Here's how the part is built. I have some questions about the finished solid (model axes, mm). Give positions to 0.01 mm unless a question says otherwise; leave off trailing zeros. Loops run counter-clockwise (first coordinate to the right, second up) from the corner with the lowest first, then second, coordinate; pieces in that order, holes last. Notation, with made-up numbers: (64, 86) - (68, 86) arc R25 ccw to (68, 98) - close; hole circle Ø10 at (28.25, -39.5). An arc over 180 degrees is marked (long way). Use a Markdown table: item, result.
from build123d import *

# Parameters (mm, degrees)
SKETCH1_W                = 50
SKETCH1_H                = 50
BOSS_EXTRUDE1_DEPTH      = 3.175
M3_CLEARANCE_HOLE1_D     = 3.2
M3_CLEARANCE_HOLE1_DEPTH = 12.4
M3_CLEARANCE_HOLE1_TIP   = 0.96137699
M3X0_5_TAPPED_HOLE1_D    = 2.5
FILLET1_R                = 3


with BuildPart() as part:
    # Sketch1 → Boss-Extrude1 (new body)
    with BuildSketch(Plane(origin=(0, 0, 0), x_dir=(1, 0, 0), z_dir=(0, 1, 0))):
        Rectangle(SKETCH1_W, SKETCH1_H)
    extrude(amount=BOSS_EXTRUDE1_DEPTH)

    # M3 Clearance Hole1
    with Locations(Plane(origin=(0, 3.175, 0), x_dir=(1, 0, 0), z_dir=(0, 1, 0))):
        with Locations((-20, 20), (20, 20), (-20, -20), (20, -20)):
            Hole(M3_CLEARANCE_HOLE1_D / 2, depth=M3_CLEARANCE_HOLE1_DEPTH)
            with Locations((0, 0, -(M3_CLEARANCE_HOLE1_DEPTH + M3_CLEARANCE_HOLE1_TIP / 2))):  # 118° drill point
                Cone(0, M3_CLEARANCE_HOLE1_D / 2, M3_CLEARANCE_HOLE1_TIP, mode=Mode.SUBTRACT)

    # M3x0.5 Tapped Hole1 (through all)
    with Locations(Plane(origin=(0, 3.175, 0), x_dir=(1, 0, 0), z_dir=(0, 1, 0))):
        with Locations((0, 15.5), (0, -15.5)):
            Hole(M3X0_5_TAPPED_HOLE1_D / 2)

    # Fillet1
    fillet1_edges = [part.edges().sort_by_distance(p)[0] for p in [
        (25, 1.5875, 25),
        (-25, 1.5875, 25),
        (-25, 1.5875, -25),
        (25, 1.5875, -25),
    ]]
    fillet(fillet1_edges, radius=FILLET1_R)


solid = part.part
(1) Suppose I cut it at B-B on x = -20. Write out the boundary of the cut face in (y, z) (3 decimals).
A:
| item | result |
|---|---|
| outline | (0, -25) - (3.175, -25) - (3.175, -21.6) - (0, -21.6) - close; (0, -18.4) - (3.175, -18.4) - (3.175, 18.4) - (0, 18.4) - close; (0, 21.6) - (3.175, 21.6) - (3.175, 25) - (0, 25) - close |
(2) Suppose I cut it at C-C on y = 1.65. Write out the boundary of the cut face in (x, z).
A:
| item | result |
|---|---|
| outline | (-25, -22) arc R3 ccw to (-22, -25) - (22, -25) arc R3 ccw to (25, -22) - (25, 22) arc R3 ccw to (22, 25) - (-22, 25) arc R3 ccw to (-25, 22) - close; hole circle Ø3.2 at (-20, -20); hole circle Ø3.2 at (-20, 20); hole circle Ø2.5 at (0, -15.5); hole circle Ø2.5 at (0, 15.5); hole circle Ø3.2 at (20, -20); hole circle Ø3.2 at (20, 20) |
(3) We'd pull the mould along X, two halves only. Please class faces 1 (the face through (-24.14, 1.61, -24.1)), 2 (the face through (24.1, 1.61, -24.14)), 3 (the face through (20.208, 1.565, -21.586)), 4 (the face through (-19.792, 1.565, -21.586)): pulls with the +X half, pulls with the -X half, needs draft (parallel to the pull), parting line crosses it, or undercut.
A:
| item | result |
|---|---|
| face 1 | pulls with the -X half |
| face 2 | pulls with the +X half |
| face 3 | undercut |
| face 4 | undercut |
(4) If I drill on line 1 (Z direction, x = 0, y = 1.9); line 2 (X direction, y = 1.2, z = 20), over which ranges is the centre line in solid material (lowest first)?
A:
| item | result |
|---|---|
| line 1 | -25 to -16.75, -14.25 to 14.25, 16.75 to 25 |
| line 2 | -25 to -21.6, -18.4 to 18.4, 21.6 to 25 |
(5) Will this pin go through, and if not, where does the flat tip stop? pin 1 (3 mm diameter, centred on x = -20, z = -20, fed in from +Y).
A:
| item | result |
|---|---|
| pin 1 | through |
(6) Suppose I cut it at A-A on z = 20. Write out the boundary of the cut face in (x, y) (3 decimals), plus the area to 3 significant figures.
A:
| item | result |
|---|---|
| outline | (-25, 0) - (-21.6, 0) - (-21.6, 3.175) - (-25, 3.175) - close; (-18.4, 0) - (18.4, 0) - (18.4, 3.175) - (-18.4, 3.175) - close; (21.6, 0) - (25, 0) - (25, 3.175) - (21.6, 3.175) - close |
| area | 138 mm2 |
